from build123d import *

# Parameters (mm, degrees)
SKETCH1_R           = 40
SKETCH1_R_2         = 30.5
BOSS_EXTRUDE1_DEPTH = 3
SKETCH2_W           = 48
SKETCH2_H           = 30
BOSS_EXTRUDE2_DEPTH = 3
SKETCH3_R           = 30.5
BOSS_EXTRUDE3_DEPTH = 3
FILLET1_R           = 3
FILLET2_R           = 3


with BuildPart() as part:
    # Sketch1 → Boss-Extrude1 (new body)
    with BuildSketch(Plane(origin=(0, 0, 0), x_dir=(1, 0, 0), z_dir=(0, 1, 0))):
        Circle(SKETCH1_R)
        Circle(SKETCH1_R_2, mode=Mode.SUBTRACT)
    extrude(amount=BOSS_EXTRUDE1_DEPTH)

    # Sketch2 → Boss-Extrude2 (add)
    with BuildSketch(Plane(origin=(0, 3, 0), x_dir=(1, 0, 0), z_dir=(0, 1, 0))):
        with Locations((59, 0)):
            Rectangle(SKETCH2_W, SKETCH2_H)
    extrude(amount=-BOSS_EXTRUDE2_DEPTH)

    # Sketch3 → Boss-Extrude3 (add)
    with BuildSketch(Plane(origin=(83, 0, 0), x_dir=(0, 0, -1), z_dir=(1, 0, 0))):
        with BuildLine():
            Line((-15, 0), (15, 0))
            Line((15, 0), (15, 58))
            ThreePointArc((15, 58), (0, 135.080992435), (-15, 58))
            Line((-15, 58), (-15, 0))
        make_face()
        with Locations((0, 95.080992435)):
            Circle(SKETCH3_R, mode=Mode.SUBTRACT)
    extrude(amount=-BOSS_EXTRUDE3_DEPTH)

    # Fillet1
    fillet1_edges = [part.edges().sort_by_distance(p)[0] for p in [
        (37.080992435, 1.5, 15),
        (37.080992435, 1.5, -15),
        (81.5, 58, 15),
        (81.5, 58, -15),
    ]]
    fillet(fillet1_edges, radius=FILLET1_R)

    # Fillet2
    fillet2_edges = [part.edges().sort_by_distance(p)[0] for p in [
        (83, 0, 0),
        (80, 3, 0),
    ]]
    fillet(fillet2_edges, radius=FILLET2_R)


solid = part.part
Work out the finished part from the listing and answer in its coordinate system (mm). A direction names the side the tool comes from. Round coordinates to 2 decimals unless told otherwise and drop trailing zeros. Write each loop counter-clockwise with the first axis right and the second up, starting at its lowest first coordinate (ties: lowest second). Pieces come first, ordered by that corner, then holes.
1) A tool of negligible diameter and unlimited length cuts with its end or side. For faces 5 (the flat face through (80, 66, -12)), 6 (the cylindrical face through (82.1, 0.86, -0.21)), 7 (the flat face through (80.5, 19.8, -15)), from which of +Z, -Z, +X, -X, +Y, -Y can it reach the whole face along a straight path? Write none if from no direction.
2) A cutting plane is placed at B-B (x = 0). Give the vertices of the cut face in (y, z), plus the area to 3 significant figures.
3) Given pin 1 Ø22 at (x, y) = (72, 15.5) entering from -Z; pin 2 Ø24 at (y, z) = (75, 6.5) entering from -X, each flat-ended and moving along its own axis, determine where each tip first touches the part or whether it passes through.
4) Straight lines are drawn through the part: line 1 (Y direction, x = -31.5, z = -7); line 2 (X direction, y = 1.3, z = 0); line 3 (X direction, y = 0.65, z = 0). For each, find the intervals that lie inside material, in ascending order.
5) A cutting plane is placed at C-C (y = 74). Give the vertices of the cut face in (x, z).
6) The mould has two halves that part along Z. Classify faces 1 (the cylindrical face through (-24.204, 1.479, 18.559)), 2 (the cylindrical face through (-39.97, 1.48, -1.52)), 3 (the cylindrical face through (79.14, 3.9, -0.21)), 4 (the flat face through (80.5, 19.8, 15)): pulls with the +Z half, pulls with the -Z half, needs draft (parallel to the pull), parting line crosses it, or undercut.
7) A cutting plane is placed at D-D (z = -23). Give the vertices of the cut face in (x, y).
8) A cutting plane is placed at A-A (z = 0). Give the vertices of the cut face in (x, y).
Completed:
1. face 5: +Z, -Z, -X, +Y
1. face 6: +Z, -Z, +X, -Y
1. face 7: -Z, +X, -Y
2. outline: (0, -40) - (3, -40) - (3, -30.5) - (0, -30.5) - close; (0, 30.5) - (3, 30.5) - (3, 40) - (0, 40) - close
2. area: 57.0 mm2
3. pin 1: stops at z = -15
3. pin 2: stops at x = 80
4. line 1: y = 0 to 3
4. line 2: x = -40 to -30.5, 30.5 to 82.47
4. line 3: x = -40 to -30.5, 30.5 to 81.86
5. outline: (80, -33.99) - (83, -33.99) - (83, -22.04) - (80, -22.04) - close; (80, 22.04) - (83, 22.04) - (83, 33.99) - (80, 33.99) - close
6. face 1: undercut
6. face 2: parting line crosses it
6. face 3: needs draft
6. face 4: pulls with the +Z half
7. outline: (-32.73, 0) - (-20.03, 0) - (-20.03, 3) - (-32.73, 3) - close; (20.03, 0) - (32.73, 0) - (32.73, 3) - (20.03, 3) - close; (80, 62.35) - (83, 62.35) - (83, 75.05) - (80, 75.05) - close; (80, 115.11) - (83, 115.11) - (83, 127.81) - (80, 127.81) - close
8. outline: (-40, 0) - (-30.5, 0) - (-30.5, 3) - (-40, 3) - close; (30.5, 0) - (80, 0) arc R3 ccw to (83, 3) - (83, 64.58) - (80, 64.58) - (80, 6) arc R3 cw to (77, 3) - (30.5, 3) - close; (80, 125.58) - (83, 125.58) - (83, 135.08) - (80, 135.08) - close
